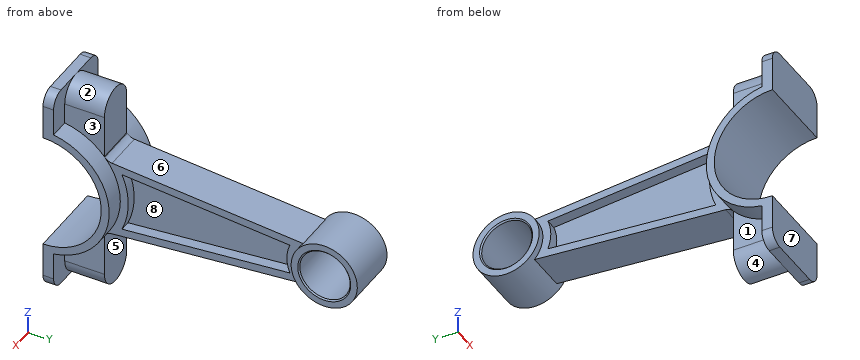
from build123d import *

# Parameters (mm, degrees)
BOSS_EXTRUDE1_DEPTH     = 15
BOSS_EXTRUDE2_DEPTH     = 7.5
SKETCH5_R               = 12.5
BOSS_EXTRUDE3_DEPTH     = 10
BOSS_EXTRUDE4_DEPTH     = 15
CUT_EXTRUDE2_DEPTH      = 126.139759491
CUT_EXTRUDE2_DEPTH_BACK = 126.139759491
SKETCH7_R               = 22
SKETCH7_R_2             = 9.5
CUT_EXTRUDE3_DEPTH      = 4
CHAMFER1_SIZE           = 0.5
FILLET1_R               = 5
FILLET2_R               = 4


with BuildPart() as part:
    # Sketch3 → Boss-Extrude1 (new, symmetric)
    with BuildSketch(Plane(origin=(0, 0, 0), x_dir=(0, 0, -1), z_dir=(1, 0, 0))):
        with BuildLine():
            Line((40, 0), (-40, 0))
            Line((-40, 0), (-40, 4))
            Line((-40, 4), (-24.677925359, 4))
            ThreePointArc((-24.677925359, 4), (0, 25), (24.677925359, 4))
            Line((24.677925359, 4), (40, 4))
            Line((40, 4), (40, 0))
        make_face()
    extrude(amount=BOSS_EXTRUDE1_DEPTH, both=True)

    # Sketch4 → Boss-Extrude2 (add, symmetric)
    with BuildSketch(Plane(origin=(0, 0, 0), x_dir=(0, 0, -1), z_dir=(1, 0, 0))):
        Polygon((7.5, 103.409272302), (16.54713903, 0), (-16.54713903, 0), (-7.5, 103.409272302), align=None)
    extrude(amount=BOSS_EXTRUDE2_DEPTH, both=True)

    # Sketch5 → Boss-Extrude3 (add, symmetric)
    with BuildSketch(Plane(origin=(0, 0, 0), x_dir=(0, 0, -1), z_dir=(1, 0, 0))):
        with Locations((0, 103.409272302)):
            Circle(SKETCH5_R)
    extrude(amount=BOSS_EXTRUDE3_DEPTH, both=True)

    # Sketch6 → Boss-Extrude4 (add)
    with BuildSketch(Plane(origin=(0, 4, 0), x_dir=(1, 0, 0), z_dir=(0, 1, 0))):
        with BuildLine():
            Line((-7.5, -32.5), (-7.5, 32.5))
            ThreePointArc((-7.5, 32.5), (0, 40), (7.5, 32.5))
            Line((7.5, 32.5), (7.5, -32.5))
            ThreePointArc((7.5, -32.5), (0, -40), (-7.5, -32.5))
        make_face()
    extrude(amount=BOSS_EXTRUDE4_DEPTH)

    # Sketch7 → Cut-Extrude2 (cut, two sides: drawn at the far end of the back side and taken through both)
    with BuildSketch(Plane(origin=(10, 0, 0), x_dir=(0, 0, -1), z_dir=(1, 0, 0)).offset(-CUT_EXTRUDE2_DEPTH_BACK)):
        Circle(SKETCH7_R)
        with Locations((0, 103.409272302)):
            Circle(SKETCH7_R_2)
    extrude(amount=CUT_EXTRUDE2_DEPTH + CUT_EXTRUDE2_DEPTH_BACK, mode=Mode.SUBTRACT)

    # Sketch13 → Cut-Extrude3 (cut)
    with BuildSketch(Plane(origin=(7.5, 0, 0), x_dir=(0, 0, -1), z_dir=(1, 0, 0))):
        with BuildLine():
            Line((-5.747925596, 89.014434639), (-11.294120161, 25.621140681))
            ThreePointArc((-11.294120161, 25.621140681), (0, 28), (11.294120161, 25.621140681))
            Line((11.294120161, 25.621140681), (5.747925596, 89.014434639))
            ThreePointArc((5.747925596, 89.014434639), (0, 87.909272302), (-5.747925596, 89.014434639))
        make_face()
    cut_extrude3 = extrude(amount=-CUT_EXTRUDE3_DEPTH, mode=Mode.SUBTRACT)

    # Mirror1: Cut-Extrude3 across plane
    add(cut_extrude3.mirror(Plane(origin=(0, 0, 0), x_dir=(0, 0, 1), z_dir=(1, 0, 0))), mode=Mode.SUBTRACT)

    # Chamfer1
    chamfer1_edges = [part.edges().sort_by_distance(p)[0] for p in [
        (10, 103.409272302, 9.5),
        (-10, 103.409272302, 9.5),
    ]]
    chamfer(chamfer1_edges, length=CHAMFER1_SIZE)

    # Fillet1
    fillet1_edges = [part.edges().sort_by_distance(p)[0] for p in [
        (15, 2, 40),
        (15, 2, -40),
        (-15, 2, -40),
        (-15, 2, 40),
    ]]
    fillet(fillet1_edges, radius=FILLET1_R)

    # Fillet2
    fillet2_edges = [part.edges().sort_by_distance(p)[0] for p in [
        (0, 20.16070078, 14.783306263),
        (0, 20.16070078, -14.783306263),
    ]]
    fillet(fillet2_edges, radius=FILLET2_R)


solid = part.part
Verification items for the finished model (mm, model axes). Face numbers are marked on the shaded views. A direction names the side the tool comes from. Give positions to 0.01 mm unless a question says otherwise; leave off trailing zeros. Loops run counter-clockwise (first coordinate to the right, second up) from the corner with the lowest first, then second, coordinate; pieces in that order, holes last.
1. Go/stop test with flat-tipped pins: P1, Ø12, axis at x = -4, y = 96, coming from the -Z side; P2, Ø1, axis at x = 0.5, y = 72.5, coming from the -Z side; P3, Ø4.5, axis at y = 12.5, z = 24, coming from the -X side; P4, Ø18, axis at y = 48, z = 5, coming from the +X side. Record where each tip stops, or that it passes through.
Derived:
P1: stops at z = -12.42
P2: stops at z = -10.25
P3: stops at x = -15
P4: stops at x = 7.5
2. Cross-section at C-C on x = 1.5. Record the cut outline in (y, z).
Derived:
outline: (0, -40) - (4, -40) - (4, -39.85) - (19, -39.85) - (19, -16.25) arc R25 ccw to (19.17, -16.05) arc R4 cw to (21.89, -14.63) - (94.08, -8.32) arc R12.5 ccw (long way) to (94.08, 8.32) - (21.89, 14.63) arc R4 cw to (19.17, 16.05) arc R25 ccw to (19, 16.25) - (19, 39.85) - (4, 39.85) - (4, 40) - (0, 40) - (0, 22) arc R22 cw to (0, -22) - close; hole circle Ø19 at (103.41, 0)
3. Tool access check on the marked faces 1, 2, 3 and 4. Record the directions out of +Z, -Z, +X, -X, +Y, -Y that give a thin tool (end or side, any length) a straight path to the whole face; none if there is none.
Derived:
face 1: -Z, -X, +Y
face 2: +Z, +Y
face 3: +Z, +X, +Y
face 4: -Z, +Y
4. Cross-section at D-D on z = -27. Record the cut outline in (x, y), and give its area (3 significant figures).
Derived:
outline: (-15, 0) - (15, 0) - (15, 4) - (7.5, 4) - (7.5, 19) - (-7.5, 19) - (-7.5, 4) - (-15, 4) - close
area: 345 mm2
5. Release check for a two-part mould opening along Y. For the marked faces 5, 6, 7 and 8 record: +Y half, -Y half, draft (parallel to the pull), parting line (faces both ways), or undercut.
Derived:
face 5: +Y half
face 6: undercut
face 7: -Y half
face 8: undercut
6. Material ranges on probe 1 along Z at (x, y) = (-1.25, 103.5); probe 2 along Y at (x, z) = (-3.25, 0); probe 3 along Y at (x, z) = (5.5, 3), recorded low to high.
Derived:
probe 1: z = -12.5 to -9.5, 9.5 to 12.5
probe 2: y = 22 to 93.91, 112.91 to 115.91
probe 3: y = 21.79 to 27.84, 88.2 to 94.4, 112.42 to 115.54
7. Cross-section at A-A on z = 0. Record the cut outline in (x, y).
Derived:
outline: (-15, 22) - (15, 22) - (15, 25) - (7.5, 25) - (7.5, 28) - (3.5, 28) - (3.5, 87.91) - (7.5, 87.91) - (7.5, 90.91) - (10, 90.91) - (10, 93.41) - (9.5, 93.91) - (-9.5, 93.91) - (-10, 93.41) - (-10, 90.91) - (-7.5, 90.91) - (-7.5, 87.91) - (-3.5, 87.91) - (-3.5, 28) - (-7.5, 28) - (-7.5, 25) - (-15, 25) - close; (-10, 113.41) - (-9.5, 112.91) - (9.5, 112.91) - (10, 113.41) - (10, 115.91) - (-10, 115.91) - close
8. Cross-section at B-B on y = 15.5. Record the cut outline in (x, z).
Derived:
outline: (-15, -19.62) - (-7.5, -19.62) - (-7.5, -32.5) arc R7.5 ccw to (7.5, -32.5) - (7.5, -19.62) - (15, -19.62) - (15, -15.61) - (-15, -15.61) - close; (-15, 15.61) - (15, 15.61) - (15, 19.62) - (7.5, 19.62) - (7.5, 32.5) arc R7.5 ccw to (-7.5, 32.5) - (-7.5, 19.62) - (-15, 19.62) - close
